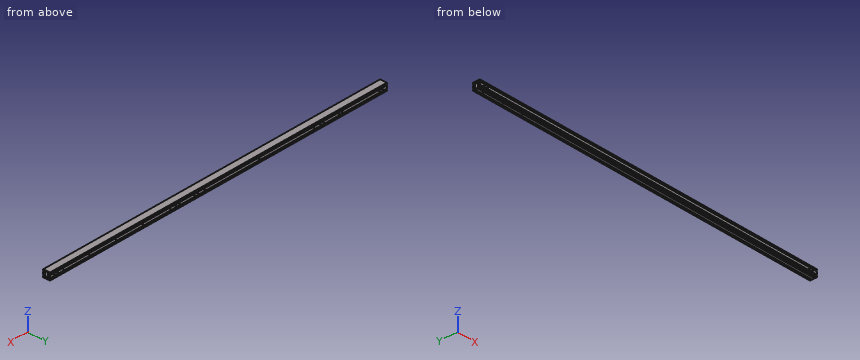
from build123d import *

# Parameters (mm, degrees)
SKETCH_1_W             = 23.5
SKETCH_1_H             = 12
EXTRUDE_1_DEPTH        = 771
HOLE_WIZARD_M6_1_D     = 5
HOLE_WIZARD_M6_1_DEPTH = 15
HOLE_WIZARD_M6_1_TIP   = 1.502151548
HOLE_WIZARD_M6_2_D     = 5
HOLE_WIZARD_M6_2_DEPTH = 15
HOLE_WIZARD_M6_2_TIP   = 1.502151548
HOLE_WIZARD_M4_1_D     = 3.3
HOLE_WIZARD_M4_1_DEPTH = 10.1
HOLE_WIZARD_M4_1_TIP   = 0.991420021
HOLE_WIZARD_M4_2_D     = 3.3
HOLE_WIZARD_M4_2_DEPTH = 10.1
HOLE_WIZARD_M4_2_TIP   = 0.991420021
HOLE_WIZARD_M6_3_D     = 5
HOLE_WIZARD_M6_3_DEPTH = 15
HOLE_WIZARD_M6_3_TIP   = 1.502151548


with BuildPart() as part:
    # 草图1 → 凸台-拉伸1 (new, symmetric)
    with BuildSketch(Plane(origin=(0, 0, 0), x_dir=(0, 0, -1), z_dir=(1, 0, 0))):
        with BuildLine():
            Line((-14, 15), (-11.5, 15))
            Line((-11.5, 15), (-11.5, 13.5))
            Line((-11.5, 13.5), (-11.4, 13.5))
            ThreePointArc((-11.4, 13.5), (-11.117157288, 13.382842712), (-11, 13.1))
            Line((-11, 13.1), (-11, 12))
            Line((-11, 12), (-9.5, 12))
            Line((-9.5, 12), (-9.5, 15))
            Line((-9.5, 15), (-8, 15))
            Line((-8, 15), (-8, 12.5))
            Line((-8, 12.5), (-5, 12.5))
            Line((-5, 12.5), (-5, 15))
            Line((-5, 15), (5, 15))
            Line((5, 15), (5, 12.5))
            Line((5, 12.5), (8, 12.5))
            Line((8, 12.5), (8, 15))
            Line((8, 15), (9.5, 15))
            Line((9.5, 15), (9.5, 12))
            Line((9.5, 12), (11, 12))
            Line((11, 12), (11, 13.1))
            ThreePointArc((11, 13.1), (11.117157288, 13.382842712), (11.4, 13.5))
            Line((11.4, 13.5), (11.5, 13.5))
            Line((11.5, 13.5), (11.5, 15))
            Line((11.5, 15), (14, 15))
            ThreePointArc((14, 15), (14.707106781, 14.707106781), (15, 14))
            Line((15, 14), (15, 8))
            Line((15, 8), (12.5, 8))
            Line((12.5, 8), (12.5, 5))
            Line((12.5, 5), (15, 5))
            Line((15, 5), (15, -5))
            Line((15, -5), (12.5, -5))
            Line((12.5, -5), (12.5, -8))
            Line((12.5, -8), (15, -8))
            Line((15, -8), (15, -14))
            ThreePointArc((15, -14), (14.707106781, -14.707106781), (14, -15))
            Line((14, -15), (11.5, -15))
            Line((11.5, -15), (11.5, -13.5))
            Line((11.5, -13.5), (11.4, -13.5))
            ThreePointArc((11.4, -13.5), (11.117157288, -13.382842712), (11, -13.1))
            Line((11, -13.1), (11, -12))
            Line((11, -12), (9.5, -12))
            Line((9.5, -12), (9.5, -15))
            Line((9.5, -15), (8, -15))
            Line((8, -15), (8, -12.5))
            Line((8, -12.5), (5, -12.5))
            Line((5, -12.5), (5, -15))
            Line((5, -15), (-5, -15))
            Line((-5, -15), (-5, -12.5))
            Line((-5, -12.5), (-8, -12.5))
            Line((-8, -12.5), (-8, -15))
            Line((-8, -15), (-9.5, -15))
            Line((-9.5, -15), (-9.5, -12))
            Line((-9.5, -12), (-11, -12))
            Line((-11, -12), (-11, -13.1))
            ThreePointArc((-11, -13.1), (-11.117157288, -13.382842712), (-11.4, -13.5))
            Line((-11.4, -13.5), (-11.5, -13.5))
            Line((-11.5, -13.5), (-11.5, -15))
            Line((-11.5, -15), (-14, -15))
            ThreePointArc((-14, -15), (-14.707106781, -14.707106781), (-15, -14))
            Line((-15, -14), (-15, 14))
            ThreePointArc((-15, 14), (-14.707106781, 14.707106781), (-14, 15))
        make_face()
        with BuildLine():
            Line((12, -10.5), (12, -8.5))
            ThreePointArc((12, -8.5), (11.853553391, -8.146446609), (11.5, -8))
            Line((11.5, -8), (-11.5, -8))
            ThreePointArc((-11.5, -8), (-11.853553391, -8.146446609), (-12, -8.5))
            Line((-12, -8.5), (-12, -10.5))
            ThreePointArc((-12, -10.5), (-11.853553391, -10.853553391), (-11.5, -11))
            Line((-11.5, -11), (11.5, -11))
            ThreePointArc((11.5, -11), (11.853553391, -10.853553391), (12, -10.5))
        make_face(mode=Mode.SUBTRACT)
        with BuildLine():
            Line((-11.5, 11), (11.5, 11))
            ThreePointArc((11.5, 11), (11.853553391, 10.853553391), (12, 10.5))
            Line((12, 10.5), (12, 8.5))
            ThreePointArc((12, 8.5), (11.853553391, 8.146446609), (11.5, 8))
            Line((11.5, 8), (-11.5, 8))
            ThreePointArc((-11.5, 8), (-11.853553391, 8.146446609), (-12, 8.5))
            Line((-12, 8.5), (-12, 10.5))
            ThreePointArc((-12, 10.5), (-11.853553391, 10.853553391), (-11.5, 11))
        make_face(mode=Mode.SUBTRACT)
        Rectangle(SKETCH_1_W, SKETCH_1_H, mode=Mode.SUBTRACT)
    extrude(amount=EXTRUDE_1_DEPTH, both=True)

    # M6 螺纹孔1
    with Locations(Plane(origin=(0, 15, 0), x_dir=(-1, 0, 0), z_dir=(0, 1, 0))):
        with Locations((-751, 0), (-736, 0), (-194, 0), (-179, 0), (-109, 0), (-94, 0), (466, 0), (481, 0), (551, 0), (566, 0), (736, 0), (751, 0)):
            Hole(HOLE_WIZARD_M6_1_D / 2, depth=HOLE_WIZARD_M6_1_DEPTH)
            with Locations((0, 0, -(HOLE_WIZARD_M6_1_DEPTH + HOLE_WIZARD_M6_1_TIP / 2))):  # 118° drill point
                Cone(0, HOLE_WIZARD_M6_1_D / 2, HOLE_WIZARD_M6_1_TIP, mode=Mode.SUBTRACT)

    # M6 螺纹孔2
    with Locations(Plane.XZ.offset(15)):
        with Locations((-751, 0), (-736, 0), (751, 0), (736, 0)):
            Hole(HOLE_WIZARD_M6_2_D / 2, depth=HOLE_WIZARD_M6_2_DEPTH)
            with Locations((0, 0, -(HOLE_WIZARD_M6_2_DEPTH + HOLE_WIZARD_M6_2_TIP / 2))):  # 118° drill point
                Cone(0, HOLE_WIZARD_M6_2_D / 2, HOLE_WIZARD_M6_2_TIP, mode=Mode.SUBTRACT)

    # M4 螺纹孔1
    with Locations(Plane(origin=(0, 15, 0), x_dir=(-1, 0, 0), z_dir=(0, 1, 0))):
        with Locations((-711, 0), (-591, 0), (-471, 0), (-346, 0), (-221, 0)):
            Hole(HOLE_WIZARD_M4_1_D / 2, depth=HOLE_WIZARD_M4_1_DEPTH)
            with Locations((0, 0, -(HOLE_WIZARD_M4_1_DEPTH + HOLE_WIZARD_M4_1_TIP / 2))):  # 118° drill point
                Cone(0, HOLE_WIZARD_M4_1_D / 2, HOLE_WIZARD_M4_1_TIP, mode=Mode.SUBTRACT)

    # M4 螺纹孔2
    with Locations(Plane(origin=(0, 0, -15), x_dir=(-1, 0, 0), z_dir=(0, 0, -1))):
        with Locations((741, 0), (651, 0), (561, 0)):
            Hole(HOLE_WIZARD_M4_2_D / 2, depth=HOLE_WIZARD_M4_2_DEPTH)
            with Locations((0, 0, -(HOLE_WIZARD_M4_2_DEPTH + HOLE_WIZARD_M4_2_TIP / 2))):  # 118° drill point
                Cone(0, HOLE_WIZARD_M4_2_D / 2, HOLE_WIZARD_M4_2_TIP, mode=Mode.SUBTRACT)

    # M6 螺纹孔3
    with Locations(Plane(origin=(0, 15, 0), x_dir=(-1, 0, 0), z_dir=(0, 1, 0))):
        with Locations((436, 0), (186, 0), (-64, 0)):
            Hole(HOLE_WIZARD_M6_3_D / 2, depth=HOLE_WIZARD_M6_3_DEPTH)
            with Locations((0, 0, -(HOLE_WIZARD_M6_3_DEPTH + HOLE_WIZARD_M6_3_TIP / 2))):  # 118° drill point
                Cone(0, HOLE_WIZARD_M6_3_D / 2, HOLE_WIZARD_M6_3_TIP, mode=Mode.SUBTRACT)


solid = part.part
Verification items for the finished model (mm, model axes). Give positions to 0.01 mm unless a question says otherwise; leave off trailing zeros.
(1) Material ranges on line 1 (Y direction, x = -508, z = 0.5); line 2 (Z direction, x = -466, y = 13.15); line 3 (Y direction, x = 389.5, z = -7.5), recorded low to high.
(2) Cross-section at A-A (x = -400.5). State how many separate pieces and enclosed holes the cut face has, plus the area to 3 significant figures.
(3) Gauge pin test, flat ends, axial feed: pin 1 (0.8 mm diameter, centred on x = -189.5, z = -10.5, fed in from +Y); pin 2 (3 mm diameter, centred on x = -186, z = 0, fed in from +Y). Record the tip position at first contact, or that the pin passes through.
Worked out:
1. line 1: y = -15 to -11, -8 to -6, 6 to 8, 11 to 15
1. line 2: z = -15 to -11, -9.5 to -8, -5 to -2.5, 2.5 to 5, 8 to 9.5, 11 to 15
1. line 3: y = -12.5 to -11, -8 to -6, 6 to 8, 11 to 12.5
2. separate pieces: 1
2. enclosed holes: 3
2. area: 407 mm2
3. pin 1: stops at y = 12
3. pin 2: stops at y = -6
